Source: CAD feature listing. Evaluate the final solid. Frame: model axes, mm. A direction names the side the tool comes from. Round coordinates to 2 decimals unless told otherwise and drop trailing zeros. Order: outer loops, then holes, each group sorted by start corner. A loop starts at its lowest first (then second) coordinate and runs counter-clockwise, first axis right, second up. Notation, with made-up numbers: (6, 55.25) -> (62, 55.25) arc R25 ccw to (62, 83.25) -> close; hole circle Ø9 at (-14.5, 88). An arc over 180 degrees is marked (long way). Answer as CSV lines item,"result". Start each with the question number.
(1) Set-up query: faces 1 (the flat face through (-37, 1, 102)), 2 (the flat face through (-3, -38, 0)). Return all of +Z, -Z, +X, -X, +Y, -Y with unobstructed straight access to the full face (end or side cutting, diameter ignored); none if empty.
(2) Section query D-D (z = 183.5). Output: boundary loops of the cut face in (x, y), plus the area to 3 significant figures.
(3) Section query A-A (x = -1.5). Output: boundary loops of the cut face in (y, z).
(4) Section query C-C (z = 157). Output: boundary loops of the cut face in (x, y).
(5) Section query B-B (y = -26.5). Output: boundary loops of the cut face in (x, z), plus the area to 3 significant figures.
(6) Line query: line 1 along Y through (x, z) = (25, 28.5); line 2 along Y through (x, z) = (-31, 199.5). Output: solid intervals per line, ascending. Write a range as from..to.
(7) Pull-direction query (Y, two-part tool) for faces 3 (the flat face through (-1, 40, 102)), 4 (the flat face through (1, -40, 83)), 5 (the flat face through (1, 37, 102)); classes: +Y half, -Y half, draft (parallel to the pull), parting line (faces both ways), or undercut.
Autodesk Inventor part; units mm, degrees
ref_plane "YZ Plane" through (0, 0, 0) normal (1, 0, 0) x (0, 1, 0)
ref_plane "XZ Plane" through (0, 0, 0) normal (0, 1, 0) x (-1, 0, 0)
ref_plane "XY Plane" through (0, 0, 0) normal (0, 0, 1) x (1, 0, 0)
sketch "Sketch1" plane through (0, 0, 0) normal (0, 0, 1) x (1, 0, 0)
  line L0 (40, -40) -> (-40, -40)
  line L1 (-40, -40) -> (-40, 40)
  line L2 (-40, 40) -> (40, 40)
  line L3 (40, 40) -> (40, -40)
  line L4 (40, -40) -> (-40, 40) construction
  line L5 (-40, -40) -> (40, 40) construction
  line L6 (-37, -37) -> (37, -37)
  line L7 (37, -37) -> (37, 37)
  line L8 (37, 37) -> (-37, 37)
  line L9 (-37, 37) -> (-37, -37)
  point P0 (0, 0)
  dimension "d0" = 80
  dimension "d1" = 80
  dimension "d2" = 3
extrude "Extrusion1" add sketch "Sketch1" along normal blind 207.6194
sketch "Sketch2" plane through (0, 0, 0) normal (1, 0, 0) x (0, 1, 0)
  line L0 (40, 0) -> (-40, 0)
  line L1 (-40, 0) -> (-40, 207.6194)
  line L2 (40, 207.6194) -> (-40, 207.6194)
  line L3 (40, 0) -> (40, 207.6194)
  line L4 (40, 207.6194) -> (-40, 169.3378)
  point P0 (0, 0)
  dimension "d5" = 25.572
extrude "Extrusion2" cut sketch "Sketch2" along normal through all both and the other way through all contours L4 L1 L2
equation "\"d3\" = Lenth"
equation "\"d5\" = Leg_cut_angle"
equation "\"Lenth\" = Leg_hight"
properties part number "TZS 0984 leg tube"
Answer block:
1,face 1,"+Z, -Z"
1,face 2,"-Z, +X, -X, +Y, -Y"
2,outline,"(-40, -10.4) -> (-37, -10.4) -> (-37, 37) -> (37, 37) -> (37, -10.4) -> (40, -10.4) -> (40, 40) -> (-40, 40) -> close"
2,area,"524 mm2"
3,outline,"(-40, 0) -> (-37, 0) -> (-37, 170.77) -> (-40, 169.34) -> close; (37, 0) -> (40, 0) -> (40, 207.62) -> (37, 206.18) -> close"
4,outline,"(-40, -40) -> (40, -40) -> (40, 40) -> (-40, 40) -> close; hole (-37, -37) -> (37, -37) -> (37, 37) -> (-37, 37) -> close"
5,outline,"(-40, 0) -> (-37, 0) -> (-37, 175.8) -> (-40, 175.8) -> close; (37, 0) -> (40, 0) -> (40, 175.8) -> (37, 175.8) -> close"
5,area,"1,050 mm2"
6,line 1,"-40..-37, 37..40"
6,line 2,"37..40"
7,face 3,"+Y half"
7,face 4,"-Y half"
7,face 5,"undercut"
